Part model, mm, in its own coordinate system. Face numbers are marked on the shaded views. A direction names the side the tool comes from. Coordinates: 2 decimals unless noted, no trailing zeros. Order: outer loops, then holes, each group sorted by start corner. A loop starts at its lowest first (then second) coordinate and runs counter-clockwise, first axis right, second up.
1) Tool access for the marked faces 4 and 5: list every direction of +Z, -Z, +X, -X, +Y, -Y with a clear straight run to the whole face (end or side of a thin tool).
2) Cut at B-B (x = 17). List the corners of the cut face in (y, z), and give its area (3 significant figures).
3) Pin check, flat tips, straight feed: pin 1 Ø15 at (y, z) = (-6.5, 1) entering from +X; pin 2 Ø1.2 at (y, z) = (0, 0) entering from -X; pin 3 Ø8 at (x, y) = (16, 12.5) entering from +Z; pin 4 Ø6 at (x, y) = (86.5, 14) entering from +Z. Stop position of each tip, or through.
4) Mould opens along Y. For the marked faces 1, 2 and 3 say: +Y half, -Y half, draft (parallel to the pull), parting line (faces both ways), or undercut.
5) Cut at A-A (x = 106). List the corners of the cut face in (y, z), and give its area (3 significant figures).
6) Wall check: L1, parallel to X at y = -13, z = -5; L2, parallel to Y at x = 30.25, z = 0; L3, parallel to Y at x = 21.5, z = 3.5. Give the ranges that are in metal, low to high.
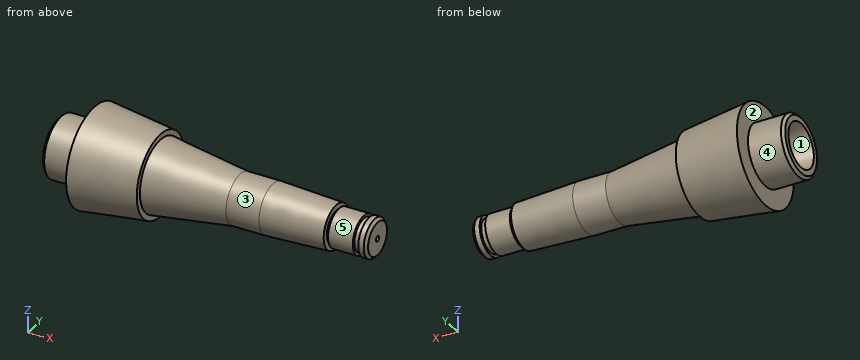
```python
from build123d import *


with BuildPart() as part:
    # Esquisse1 → Révolution1 (revolve)
    with BuildSketch(Plane.XY, mode=Mode.PRIVATE) as r_volution1_sk:
        Polygon((116, 6), (115, 7), (113, 7), (113, 6), (111, 6), (111, 7), (102, 7), (102, 6), (101, 6), (101, 8), (78, 9), (66, 9), (37, 13.055520556), (37, 15.055520556), (13, 18.055520556), (13, 11.055520556), (1, 11.055520556), (0, 10.055520556), (0, 8.055520556), (23, 4), (33, 4), (36, 1), (65, 1), (66, 0.5), (78.5, 0.5), (78.5, 0.75), (79, 0.75), (79, 1), (116, 1), align=None)
    revolve(r_volution1_sk.sketch.rotate(Axis((15.989172968, 0, 0), (-1, 0, 0)), 90), axis=Axis((15.989172968, 0, 0), (-1, 0, 0)))


solid = part.part
```
Geometry check:
1. face 4: -X
1. face 5: +X
2. outline: circle Ø35.11 at (0, 0); hole circle Ø10.12 at (0, 0)
2. area: 888 mm2
3. pin 1: stops at x = 116
3. pin 2: stops at x = 65.8
3. pin 3: stops at z = 15.58
3. pin 4: passes through
4. face 1: undercut
4. face 2: draft
4. face 3: parting line
5. outline: circle Ø14 at (0, 0); hole circle Ø2 at (0, 0)
5. area: 151 mm2
6. L1: x = 13 to 37
6. L2: y = -15.9 to -4, 4 to 15.9
6. L3: y = -16.63 to -2.44, 2.44 to 16.63
